Here's the drawing with two shaded views (mm, measured from the low corner). I have some questions. A direction names the side the tool comes from. Round coordinates to 2 decimals unless told otherwise and drop trailing zeros. Loops run counter-clockwise (first coordinate to the right, second up) from the corner with the lowest first, then second, coordinate; pieces in that order, holes last. Notation, with made-up numbers: (45, -21) -> (96, -21) arc R5 ccw to (96, -16) -> close; hole circle Ø7 at (16.25, 56.25). An arc over 180 degrees is marked (long way). One line per item, written item: value. Start each with the question number.
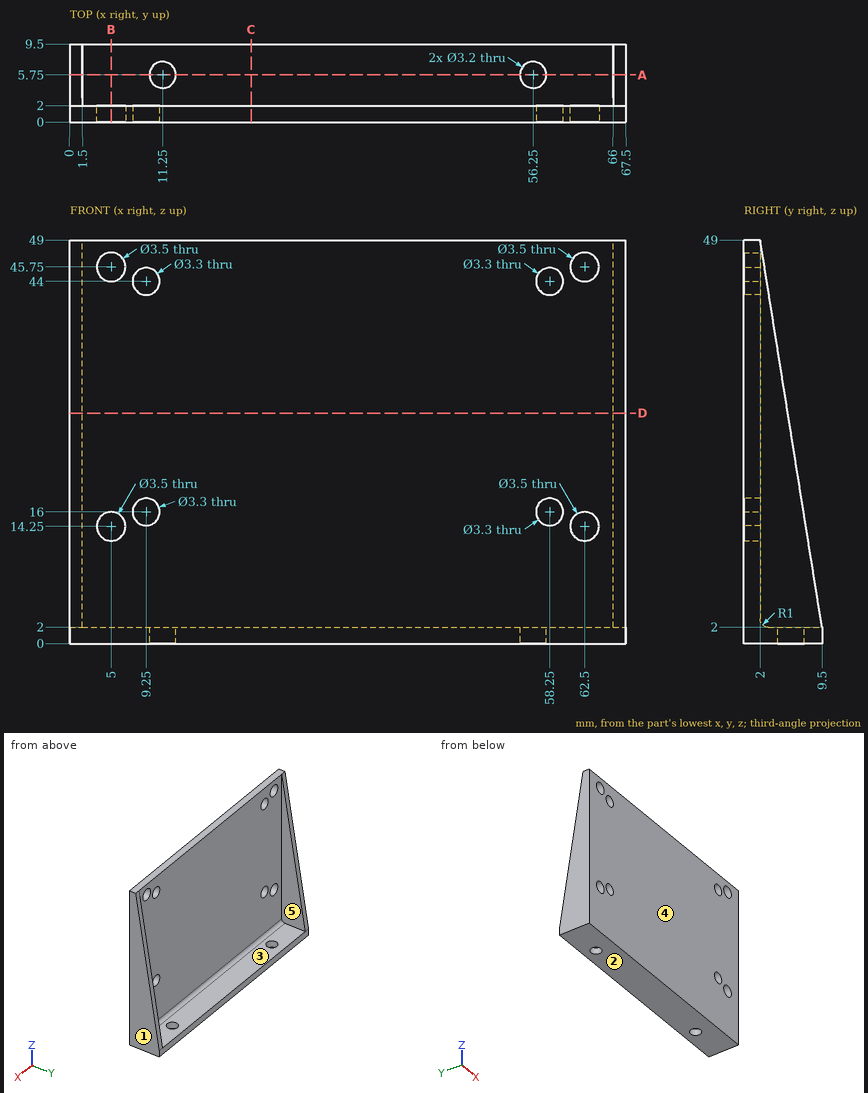
Q1. Will these pins go through, and if not, where does the flat tip stop? P1, Ø4.5, axis at x = 9.25, z = 44, coming from the +Y side; P2, Ø1, axis at x = 18, y = 6, coming from the +Z side.
Q2. If we mould it in two halves opening along X, with no side actions, what happens to the marked faces 1, 2 and 3? For each: released by +X, released by -X, zero draft, split by the parting line, or undercut.
Q3. I want a section at A-A on y = 5.75. Please give me the cut outline in (x, z), plus the area to 3 significant figures.
Q4. If I drill on line 1 along Z through (x, y) = (62.5, 0.55); line 2 along Z through (x, y) = (9.25, 1.35); line 3 along X through (y, z) = (7.5, 9), over which ranges is the centre line in solid material (lowest first)?
Q5. I want a section at D-D on z = 28. Please give me the cut outline in (x, y).
Q6. I want a section at C-C on x = 22. Please give me the cut outline in (y, z).
Q7. Which directions (+Z, -Z, +X, -X, +Y, -Y) give clear straight access to the entire face, cutting with the end or side of a thin tool? Please do the marked faces 4 and 5.
Q8. I want a section at B-B on x = 5. Please give me the cut outline in (y, z), plus the area to 3 significant figures.
Answers below:
1. P1: stops at y = 2
1. P2: stops at z = 2
2. face 1: released by +X
2. face 2: zero draft
2. face 3: undercut
3. outline: (0, 0) -> (9.65, 0) -> (9.65, 2) -> (1.5, 2) -> (1.5, 25.5) -> (0, 25.5) -> close; (12.85, 0) -> (54.65, 0) -> (54.65, 2) -> (12.85, 2) -> close; (57.85, 0) -> (67.5, 0) -> (67.5, 25.5) -> (66, 25.5) -> (66, 2) -> (57.85, 2) -> close
3. area: 193 mm^2
4. line 1: z = 0 to 12.5, 16 to 44, 47.5 to 49
4. line 2: z = 0 to 14.35, 17.65 to 42.35, 45.65 to 49
4. line 3: x = 0 to 1.5, 66 to 67.5
5. outline: (0, 0) -> (67.5, 0) -> (67.5, 5.35) -> (66, 5.35) -> (66, 2) -> (1.5, 2) -> (1.5, 5.35) -> (0, 5.35) -> close
6. outline: (0, 0) -> (9.5, 0) -> (9.5, 2) -> (3, 2) arc R1 cw to (2, 3) -> (2, 49) -> (0, 49) -> close
7. face 4: +Z, -Z, +X, -X, -Y
7. face 5: +Z, +Y
8. outline: (0, 0) -> (9.5, 0) -> (9.5, 2) -> (3, 2) arc R1 cw to (2, 3) -> (2, 12.5) -> (0, 12.5) -> close; (0, 16) -> (2, 16) -> (2, 44) -> (0, 44) -> close; (0, 47.5) -> (2, 47.5) -> (2, 49) -> (0, 49) -> close
8. area: 99.2 mm^2
